from build123d import *

# Parameters (mm, degrees)
CHAMFER1_SIZE      = 0.375
CUT_EXTRUDE2_DEPTH = 1.19


with BuildPart() as part:
    # Sketch1 → Revolve1 (revolve)
    with BuildSketch(Plane(origin=(0, 0, 0), x_dir=(0, 0, -1), z_dir=(1, 0, 0)), mode=Mode.PRIVATE) as revolve1_sk:
        Polygon((-3.3, 1.5), (5, 1.5), (5, 0), (-3.81, 0), (-3.81, 1.5), align=None)
    revolve(revolve1_sk.sketch.rotate(Axis((0, 0, 3.81), (0, 0, -1)), 180), axis=Axis((0, 0, 3.81), (0, 0, -1)))

    # Chamfer1
    chamfer1_edges = [part.edges().sort_by_distance(p)[0] for p in [
        (0, 1.5, -5),
    ]]
    chamfer(chamfer1_edges, length=CHAMFER1_SIZE)


with BuildPart() as body_2:
    # Sketch7 → Revolve2 (revolve)
    with BuildSketch(Plane(origin=(0, 0, 0), x_dir=(0, 0, -1), z_dir=(1, 0, 0)), mode=Mode.PRIVATE) as revolve2_sk:
        Polygon((-5, 3), (-4.915, 3), (-3.3, 1.385), (-3.3, 0), (-5, 0), align=None)
    revolve(revolve2_sk.sketch.rotate(Axis((0, 0, 5), (0, 0, -1)), 180), axis=Axis((0, 0, 5), (0, 0, -1)))

    # Sketch5 → Cut-Extrude2 (cut)
    with BuildSketch(Plane.XY.offset(5)):
        Polygon((1, -0.577350269), (1, 0.577350269), (0, 1.154700538), (-1, 0.577350269), (-1, -0.577350269), (0, -1.154700538), align=None)
    extrude(amount=-CUT_EXTRUDE2_DEPTH, mode=Mode.SUBTRACT)

    # Cut-Extrude3 cone 1 section (through the dimple's axis) → Cut-Extrude3 (revolve, cut)
    with BuildSketch(Plane(origin=(0, 0, 5), x_dir=(0, -1, 0), z_dir=(1, 0, 0))):
        Polygon((0, 0), (1.154700538, 0), (0, 1.154700538), align=None)
    revolve(axis=Axis((0, 0, 5), (0, 0, -1)), mode=Mode.SUBTRACT)

    # Combine1: union part
    add(part.part)


solid = body_2.part
Geometry check sheet. Reference: the model listing, model coordinates, mm. A direction names the side the tool comes from. Give positions to 0.01 mm unless a question says otherwise; leave off trailing zeros. Loops run counter-clockwise (first coordinate to the right, second up) from the corner with the lowest first, then second, coordinate; pieces in that order, holes last. Notation, with made-up numbers: M 0,-39 L 17,-39 A23 cw 17,-19 Z; hole C 52.5,71.25 d9. An arc over 180 degrees is marked long. Write each question's results on one line, items separated by ' | '.
1) Section check A-A, the plane y = 0. Record the boundary of the cut face in (x, z) (3 decimals), plus the area to 3 significant figures.
Answers follow:
outline: M -3,4.915 L -1.5,3.415 L -1.5,-4.625 L -1.125,-5 L 1.125,-5 L 1.5,-4.625 L 1.5,3.415 L 3,4.915 L 3,5 L 1.155,5 L 1,4.845 L 1,3.81 L -1,3.81 L -1,4.845 L -1.155,5 L -3,5 Z | area: 30.0 mm2
2) Thickness scan on line 1 (Z direction, x = 0.1, y = 0.25); line 2 (Y direction, x = 0.05, z = -0.5); line 3 (Y direction, x = 0.55, z = 4.75). Record the ranges inside material, lowest first.
Answers follow:
line 1: -5 to 3.81 | line 2: -1.5 to 1.5 | line 3: -2.78 to -0.84, 0.84 to 2.78
3) Release check for a two-part mould opening along Y. For faces 1 (the face through (-0.49, 0.87, 4.41)), 2 (the face through (-0.45, -1.43, -0.55)), 3 (the face through (0, 0, -5)) record: +Y half, -Y half, draft (parallel to the pull), parting line (faces both ways), or undercut.
Answers follow:
face 1: undercut | face 2: parting line | face 3: draft
4) Gauge pin test, flat ends, axial feed: pin 1 (0.6 mm diameter, centred on y = -0.5, z = 4, fed in from -X); pin 2 (3 mm diameter, centred on y = -2, z = 3, fed in from -X). Record the tip position at first contact, or that the pin passes through.
Answers follow:
pin 1: x = -2.34 | pin 2: x = -2.03
5) Tool access check on faces 4 (the face through (1, 1, 5)), 5 (the face through (-0.51, -0.86, 4.41)). Record the directions out of +Z, -Z, +X, -X, +Y, -Y that give a thin tool (end or side, any length) a straight path to the whole face; none if there is none.
Answers follow:
face 4: +Z, +X, -X, +Y, -Y | face 5: +Z
6) Section check B-B, the plane z = 0. Record the boundary of the cut face in (x, y), plus the area to 3 significant figures.
Answers follow:
outline: C 0,0 d3 | area: 7.07 mm2
